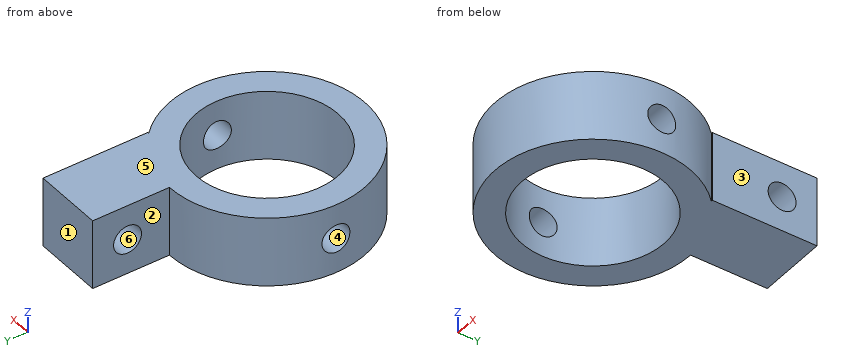
from build123d import *

# Parameters (mm, degrees)
CYLINDER003_R           = 2
CYLINDER003_DEPTH       = 10
CYLINDER003_PITCH_ANGLE = -90
CYLINDER004_R           = 2
CYLINDER004_DEPTH       = 30
CYLINDER004_PITCH_ANGLE = -90
CYLINDER001_R           = 10.2
CYLINDER001_DEPTH       = 10
BOX_W                   = 10
BOX_H                   = 15
BOX_DEPTH               = 10
CYLINDER_R              = 14
CYLINDER_DEPTH          = 10


with BuildPart() as cylinder003:
    # Cylinder003 → Cylinder003 (new body)
    with BuildSketch(Plane.XY):
        Circle(CYLINDER003_R)
    extrude(amount=CYLINDER003_DEPTH)


with BuildPart() as cylinder003_1:
    # Cylinder003 pitch: moved
    add(cylinder003.part.rotate(Axis((0, 0, 0), (0, 1, 0)), CYLINDER003_PITCH_ANGLE))


with BuildPart() as cylinder003_2:
    # Cylinder003 placement: moved
    add(cylinder003_1.part.moved(Location((10, 20, 0))))


with BuildPart() as cylinder004:
    # Cylinder004 → Cylinder004 (new body)
    with BuildSketch(Plane.XY):
        Circle(CYLINDER004_R)
    extrude(amount=CYLINDER004_DEPTH)


with BuildPart() as cylinder004_1:
    # Cylinder004 pitch: moved
    add(cylinder004.part.rotate(Axis((0, 0, 0), (0, 1, 0)), CYLINDER004_PITCH_ANGLE))


with BuildPart() as cylinder004_2:
    # Cylinder004 placement: moved
    add(cylinder004_1.part.moved(Location((15, 0, 0))))


with BuildPart() as negative_fusion:
    # Cylinder001 → Cylinder001 (new body)
    with BuildSketch(Plane.XY.offset(-5)):
        Circle(CYLINDER001_R)
    extrude(amount=CYLINDER001_DEPTH)

    # Fusion: union Cylinder003, Cylinder004
    add(cylinder003_2.part)
    add(cylinder004_2.part)


with BuildPart() as cube:
    # Box → Box (new body)
    with BuildSketch(Plane(origin=(0, 10, -5), x_dir=(1, 0, 0), z_dir=(0, 0, 1))):
        with Locations((5, 7.5)):
            Rectangle(BOX_W, BOX_H)
    extrude(amount=BOX_DEPTH)


with BuildPart() as cut:
    # Cylinder → Cylinder (new body)
    with BuildSketch(Plane.XY.offset(-5)):
        Circle(CYLINDER_R)
    extrude(amount=CYLINDER_DEPTH)

    # Fusion001: union Cube
    add(cube.part)

    # Cut: cut Negative Fusion
    add(negative_fusion.part, mode=Mode.SUBTRACT)


solid = cut.part
Part model, mm, in its own coordinate system. Face numbers are marked on the shaded views. A direction names the side the tool comes from. Coordinates: 2 decimals unless noted, no trailing zeros. Loops run counter-clockwise (first coordinate to the right, second up) from the corner with the lowest first, then second, coordinate; pieces in that order, holes last. Notation, with made-up numbers: M 56,34 L 83,34 A26 ccw 83,64 Z; hole C 45.25,47.5 d3. An arc over 180 degrees is marked long. Use a Markdown table: item, result. Add a question column.
Q1. Cut at C-C (x = -4.5). Write the cut outline in (y, z), and give its area (3 significant figures).
Q2. Probe L1, parallel to Z at x = -11.6, y = 0; L2, parallel to Y at x = 1.75, z = 0.75; L3, parallel to Y at x = 4.5, z = -1. List the from-to ranges inside material, lowest first.
Q3. Cut at D-D (y = 20). Write the cut outline in (x, z), and give its area (3 significant figures).
Q4. Cut at A-A (y = 0). Write the cut outline in (x, z).
Q5. Cut at B-B (z = 0). Write the cut outline in (x, y).
Q6. Pin check, flat tips, straight feed: P1, Ø2.5, axis at y = 0, z = 0, coming from the +X side; P2, Ø1, axis at y = -3.5, z = 2, coming from the +X side; P3, Ø5, axis at y = 18, z = -2.5, coming from the +X side; P4, Ø3, axis at y = 20, z = 2, coming from the -X side. Stop position of each tip, or through.
Q7. Mould opens along Z. For the marked faces 3, 4, 5 and 6 say: +Z half, -Z half, draft (parallel to the pull), parting line (faces both ways), or undercut.
Q8. Which spindle directions (+Z, -Z, +X, -X, +Y, -Y) get a long thin tool onto all of the face, cutting with end or side? Do the marked faces 1 and 2. Say none if no direction does.
Worked out:
| question | item | result |
|---|---|---|
| 1 | outline | M -13.26,-5 L -9.15,-5 L -9.15,5 L -13.26,5 Z; M 9.15,-5 L 13.26,-5 L 13.26,5 L 9.15,5 Z |
| 1 | area | 82.1 mm2 |
| 2 | L1 | z = -5 to -2, 2 to 5 |
| 2 | L2 | y = -13.89 to -10.05, 10.05 to 18.15, 21.85 to 25 |
| 2 | L3 | y = -13.26 to -9.15, 9.15 to 18.27, 21.73 to 25 |
| 3 | outline | M 0,-5 L 10,-5 L 10,-2 L 0,-2 Z; M 0,2 L 10,2 L 10,5 L 0,5 Z |
| 3 | area | 60.0 mm2 |
| 4 | outline | M -14,-5 L -10.2,-5 L -10.2,-2 L -14,-2 Z; M -14,2 L -10.2,2 L -10.2,5 L -14,5 Z; M 10.2,-5 L 14,-5 L 14,-2 L 10.2,-2 Z; M 10.2,2 L 14,2 L 14,5 L 10.2,5 Z |
| 5 | outline | M -13.86,-2 A14 ccw 13.86,-2 L 10,-2 A10.2 cw -10,-2 Z; M -13.86,2 L -10,2 A10.2 cw 10,2 L 13.86,2 A14 ccw 9.8,10 L 10,10 L 10,18 L 0,18 L 0,14 A14 ccw Z; M 0,22 L 10,22 L 10,25 L 0,25 Z |
| 6 | P1 | passes through |
| 6 | P2 | stops at x = 13.67 |
| 6 | P3 | stops at x = 10 |
| 6 | P4 | stops at x = 0 |
| 7 | face 3 | draft |
| 7 | face 4 | undercut |
| 7 | face 5 | +Z half |
| 7 | face 6 | undercut |
| 8 | face 1 | +Z, -Z, +X, -X, +Y |
| 8 | face 2 | +Z, -Z, -X, +Y |
